```python
from build123d import *

# Parameters (mm, degrees)
ESBO_O1_R             = 6
EXTRUS_O1_DEPTH       = 40
ESBO_O2_R             = 5
CORTE_EXTRUS_O1_DEPTH = 30
CHANFRO1_SIZE         = 0.5
ESBO_O3_W             = 3
ESBO_O3_H             = 2


with BuildPart() as part:
    # Esboço1 → Extrusão1 (new body)
    with BuildSketch(Plane(origin=(0, 0, 0), x_dir=(1, 0, 0), z_dir=(0, 1, 0))):
        with Locations(Location((0, 0, 0), (0, 0, 270))):  # turned: the seam where the file's is
            Circle(ESBO_O1_R)
    extrude(amount=EXTRUS_O1_DEPTH)

    # Esboço2 → Corte-extrusão1 (cut)
    with BuildSketch(Plane.XZ):
        with Locations(Location((0, 0, 0), (0, 0, 270))):  # turned: the seam where the file's is
            Circle(ESBO_O2_R)
    extrude(amount=-CORTE_EXTRUS_O1_DEPTH, mode=Mode.SUBTRACT)

    # Chanfro1
    chanfro1_edges = [part.edges().sort_by_distance(p)[0] for p in [
        (0, 40, -6),
    ]]
    chamfer(chanfro1_edges, length=CHANFRO1_SIZE)

    # Esboço3 → Corte-Revolução3 (revolve, cut)
    with BuildSketch(Plane.XY, mode=Mode.PRIVATE) as corte_revolu_o3_sk:
        with Locations((6.5, 35)):
            Rectangle(ESBO_O3_W, ESBO_O3_H)
    revolve(corte_revolu_o3_sk.sketch.rotate(Axis((0, 0, 0), (0, 1, 0)), 90), axis=Axis((0, 0, 0), (0, 1, 0)), mode=Mode.SUBTRACT)  # turned: the seam where the file's is


solid = part.part
```
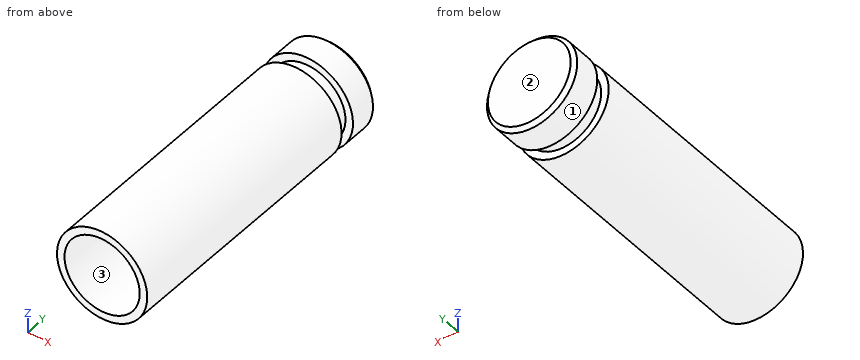
Can you work these out from the model? Positions are in its coordinate system, mm. Face numbers are marked on the shaded views. Give positions to 0.01 mm unless a question says otherwise; leave off trailing zeros. Loops run counter-clockwise (first coordinate to the right, second up) from the corner with the lowest first, then second, coordinate; pieces in that order, holes last. Notation, with made-up numbers: M 61.25,-31 L 104.25,-31 A19 ccw 104.25,-13 Z; hole C -32,-31 d7. An arc over 180 degrees is marked long. One line per question, with ' | ' between items. Start each with the question number.
Q1. If we section it at D-D (y = 33): Please give me the cut outline in (x, z), plus the area to 3 significant figures.
Q2. If we section it at A-A (x = 0): Please give me the cut outline in (y, z).
Q3. If I drill on line 1 (X direction, y = 10.5, z = 0); line 2 (Y direction, x = 3.5, z = -2.5); line 3 (Y direction, x = 1, z = 5.25), over which ranges is the centre line in solid material (lowest first)? Write a range as from..to.
Q4. If we section it at C-C (y = 9.5): Please give me the cut outline in (x, z).
Q5. If we mould it in two halves opening along Z, with no side actions, what happens to the marked faces 1, 2 and 3? For each: +Z half, -Z half, draft (parallel to the pull), parting line (faces both ways), or undercut.
Q6. For pin 1 Ø3.5 at (x, z) = (-0.5, 0.5) entering from -Y; pin 2 Ø5 at (x, y) = (-5, 29.5) entering from -Z; pin 3 Ø1 at (x, y) = (4.5, 19.5) entering from -Z; pin 4 Ø4 at (x, z) = (4.5, 0.5) entering from -Y, each with a flat end and sliding along its axis, tell me the tip position at first contact or that it passes through.
Q7. If we section it at B-B (z = 0): Please give me the cut outline in (x, y).
Computed:
1) outline: C 0,0 d12 | area: 113 mm²
2) outline: M 0,-6 L 34,-6 L 34,-5 L 36,-5 L 36,-6 L 39.5,-6 L 40,-5.5 L 40,5.5 L 39.5,6 L 36,6 L 36,5 L 34,5 L 34,6 L 0,6 L 0,5 L 30,5 L 30,-5 L 0,-5 Z
3) line 1: x = -6..-5, 5..6 | line 2: y = 30..40 | line 3: y = 0..34, 36..40
4) outline: C 0,0 d12; hole C 0,0 d10
5) face 1: parting line | face 2: draft | face 3: undercut
6) pin 1: stops at y = 30 | pin 2: stops at z = -5.45 | pin 3: stops at z = -4.47 | pin 4: stops at y = 0
7) outline: M -6,0 L -5,0 L -5,30 L 5,30 L 5,0 L 6,0 L 6,34 L 5,34 L 5,36 L 6,36 L 6,39.5 L 5.5,40 L -5.5,40 L -6,39.5 L -6,36 L -5,36 L -5,34 L -6,34 Z
